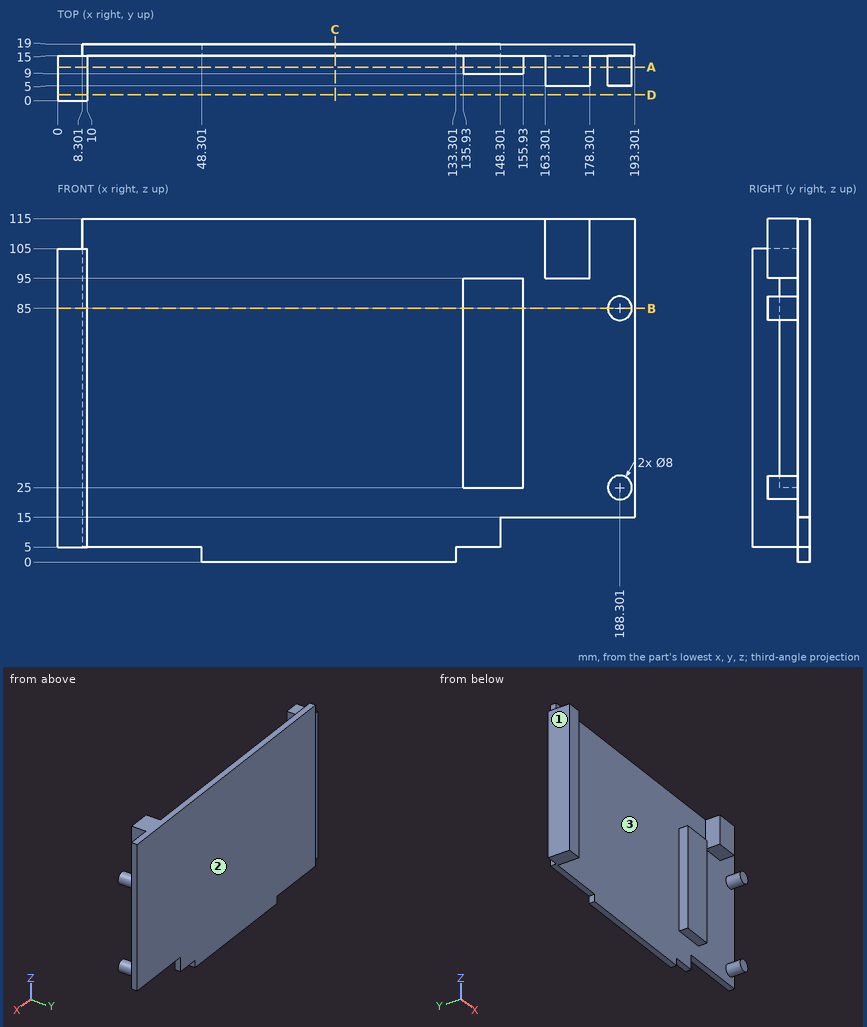
Source: three-view drawing plus pictorial views. Frame: mm from the lowest corner of the part. Round coordinates to 2 decimals unless told otherwise and drop trailing zeros. Loops run counter-clockwise (first coordinate to the right, second up) from the corner with the lowest first, then second, coordinate; pieces in that order, holes last. Notation, with made-up numbers: (32, -31) -> (39, -31) arc R20 cw to (39, 2) -> close; hole circle Ø6 at (-6.5, -2.5). An arc over 180 degrees is marked (long way). Use one line per item in the form item = value.
Item 1: Cut plane D-D on y = 2. Output: boundary loops of the cut face in (x, z).
Evaluation:
outline = (0, 5) -> (10, 5) -> (10, 105) -> (0, 105) -> close
Item 2: Contact query for flat-ended pins moving along their axis: pin 1 Ø6.5 at (x, y) = (148, 11.5) entering from -Z; pin 2 Ø4 at (y, z) = (14.5, 58.5) entering from -X; pin 3 Ø6 at (x, z) = (152, 32) entering from -Y; pin 4 Ø2.5 at (x, z) = (6, 73.5) entering from +Y. Output: stop coordinate, or through.
Evaluation:
pin_1 = 25
pin_2 = 0
pin_3 = 9
pin_4 = 15
Item 3: Draft query along X for the marked faces 1, 2 and 3. Return one class per face: released by +X, released by -X, zero draft, split by the parting line, or undercut.
Evaluation:
face_1 = released by -X
face_2 = zero draft
face_3 = undercut
Item 4: Cut plane C-C on x = 93. Output: boundary loops of the cut face in (y, z).
Evaluation:
outline = (15, 0) -> (19, 0) -> (19, 115) -> (15, 115) -> close
Item 5: Material intervals for probe 1 along X at (y, z) = (12.25, 98); probe 2 along X at (y, z) = (18, 68); probe 3 along Y at (x, z) = (139, 93), sorted ascending.
Evaluation:
probe_1 = 0 to 10, 163.3 to 178.3
probe_2 = 8.3 to 193.3
probe_3 = 9 to 19
Item 6: Cut plane B-B on z = 85. Output: boundary loops of the cut face in (x, y).
Evaluation:
outline = (0, 0) -> (10, 0) -> (10, 15) -> (135.93, 15) -> (135.93, 9) -> (155.93, 9) -> (155.93, 15) -> (184.3, 15) -> (184.3, 5) -> (192.3, 5) -> (192.3, 15) -> (193.3, 15) -> (193.3, 19) -> (8.3, 19) -> (8.3, 15) -> (0, 15) -> close
Item 7: Cut plane A-A on y = 11.25. Output: boundary loops of the cut face in (x, z).
Evaluation:
outline = (0, 5) -> (10, 5) -> (10, 105) -> (0, 105) -> close; (135.93, 25) -> (155.93, 25) -> (155.93, 95) -> (135.93, 95) -> close; (163.3, 95) -> (178.3, 95) -> (178.3, 115) -> (163.3, 115) -> close; circle Ø8 at (188.3, 25); circle Ø8 at (188.3, 85)
